Geometry: see drawing. Coordinates: mm, zero at the bounding-box minimum. Give positions to 0.01 mm unless a question says otherwise; leave off trailing zeros. Write each loop counter-clockwise with the first axis right and the second up, starting at its lowest first coordinate (ties: lowest second). Pieces come first, ordered by that corner, then holes. Notation, with made-up numbers: (-21, -19) - (14, -19) arc R23 cw to (14, 12) - close; hole circle Ø7 at (48, 88). An arc over 180 degrees is marked (long way). Use a Markdown table: item, result. Add a question column.
1. Material intervals for probe 1 along Y at (x, z) = (215, 3.1); probe 2 along Y at (x, z) = (15, 3.95); probe 3 along X at (y, z) = (17, 2.7), sorted ascending.
2. Section query C-C, the plane y = 60. Return loops of the section in (x, z), plus the area to 3 significant figures.
3. Section query A-A, the plane y = 150. Return loops of the section in (x, z), plus the area to 3 significant figures.
4. Pin query (flat end, axial travel): pin 1 (5 mm diameter, centred on x = 215, y = 60, fed in from +Z). Return the tip coordinate at first contact, or that it passes through.
5. Section query B-B, the plane x = 117.5. Return loops of the section in (y, z).
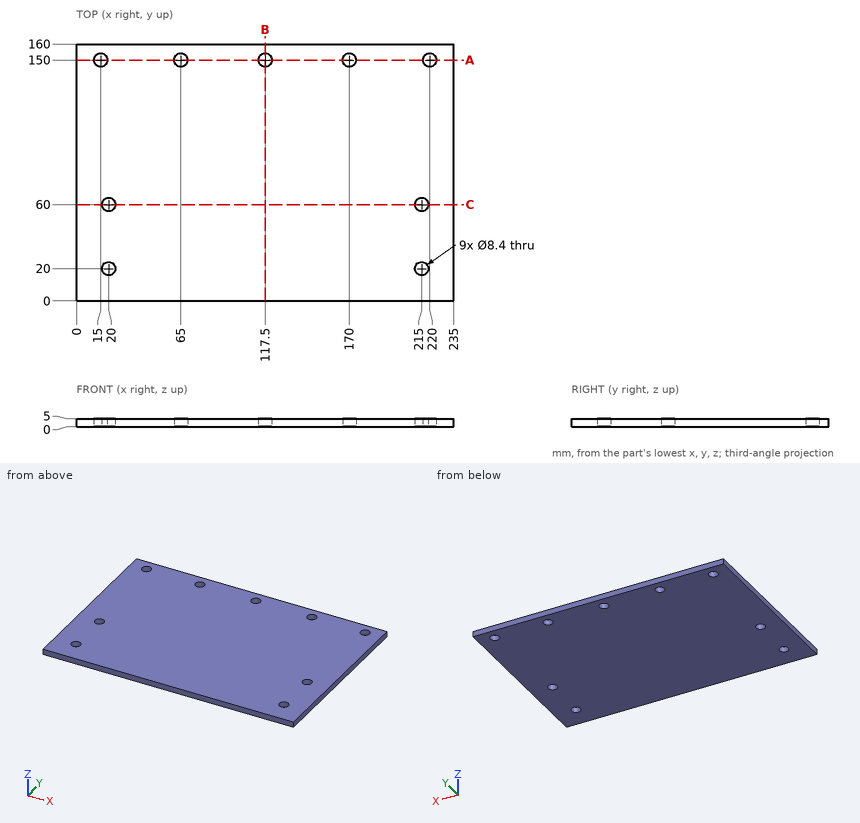
Result sheet:
| question | item | result |
|---|---|---|
| 1 | probe 1 | y = 0 to 15.8, 24.2 to 55.8, 64.2 to 160 |
| 1 | probe 2 | y = 0 to 145.8, 154.2 to 160 |
| 1 | probe 3 | x = 0 to 17.06, 22.94 to 212.06, 217.94 to 235 |
| 2 | outline | (0, 0) - (15.8, 0) - (15.8, 5) - (0, 5) - close; (24.2, 0) - (210.8, 0) - (210.8, 5) - (24.2, 5) - close; (219.2, 0) - (235, 0) - (235, 5) - (219.2, 5) - close |
| 2 | area | 1,090 mm² |
| 3 | outline | (0, 0) - (10.8, 0) - (10.8, 5) - (0, 5) - close; (19.2, 0) - (60.8, 0) - (60.8, 5) - (19.2, 5) - close; (69.2, 0) - (113.3, 0) - (113.3, 5) - (69.2, 5) - close; (121.7, 0) - (165.8, 0) - (165.8, 5) - (121.7, 5) - close; (174.2, 0) - (215.8, 0) - (215.8, 5) - (174.2, 5) - close; (224.2, 0) - (235, 0) - (235, 5) - (224.2, 5) - close |
| 3 | area | 965 mm² |
| 4 | pin 1 | passes through |
| 5 | outline | (0, 0) - (145.8, 0) - (145.8, 5) - (0, 5) - close; (154.2, 0) - (160, 0) - (160, 5) - (154.2, 5) - close |
